```python
from build123d import *

# Parameters (mm, degrees)
SALIENTE_EXTRUIR1_DEPTH = 1
CORTAR_EXTRUIR1_DEPTH   = 0.5
SALIENTE_EXTRUIR2_DEPTH = 0.5


with BuildPart() as part:
    # Croquis1 → Saliente-Extruir1 (new body)
    with BuildSketch(Plane.XY):
        Polygon((0.027506267, 9.99996217), (-9.502029281, 3.116318268), (-5.900083324, -8.073971561), (5.85557725, -8.106307117), (9.519029089, 3.063998239), align=None)
    extrude(amount=SALIENTE_EXTRUIR1_DEPTH)

    # Croquis2 → Cortar-Extruir1 (cut)
    with BuildSketch(Plane.XY.offset(1)):
        Polygon((0.042555256, 9.600245361), (-9.117225611, 3.00711142), (-5.677310567, -7.741748295), (5.608454716, -7.791774999), (9.143526206, 2.926166513), align=None)
    extrude(amount=-CORTAR_EXTRUIR1_DEPTH, mode=Mode.SUBTRACT)

    # Croquis3 → Saliente-Extruir2 (add)
    with BuildSketch(Plane.XY.offset(0.5)):
        Polygon((-5.900083324, -8.073971561), (-0.010506459, -3.819645663), (5.85557725, -8.106307117), (3.629452223, -1.190327659), (9.519029089, 3.063998239), (2.253631293, 3.083982712), (0.027506267, 9.99996217), (-2.236631486, 3.096333795), (-9.502029281, 3.116318268), (-3.635945572, -1.170343186), align=None)
    extrude(amount=SALIENTE_EXTRUIR2_DEPTH)


solid = part.part
```
Check sheet for the modelled part. Datum: model origin and axes. Units: mm. A direction names the side the tool comes from. Coordinates: 2 decimals unless noted, no trailing zeros. Order: outer loops, then holes, each group sorted by start corner. A loop starts at its lowest first (then second) coordinate and runs counter-clockwise, first axis right, second up. Notation, with made-up numbers: (6.25, -13) -> (14.25, -13) arc R19 ccw to (14.25, 5) -> close; hole circle Ø5 at (-10.5, 47.5). An arc over 180 degrees is marked (long way). Write each question's results on one line, items separated by ' | '. Start each with the question number.
1) Section check A-A (z = 0.85). Enter the section's corners in (x, y), and give its area (3 significant figures).
2) Set-up check for faces 5 (the face through (-7.726, -2.4, 0.493)), 6 (the face through (0, -6, 0.5)): record each of +Z, -Z, +X, -X, +Y, -Y from which the full face is reachable in a straight line by a thin tool's end or side.
3) Section check B-B (x = 1.25). Enter the section's corners in (y, z), and give its area (3 significant figures).
4) Material ranges on line 1 along X through (y, z) = (8.75, 0.55); line 2 along X through (y, z) = (-6, 0.8); line 3 along Y through (x, z) = (-3, 0.9), recorded low to high.
5) Depth check by flat-ended pin: pin 1 (2 mm diameter, centred on x = 0, y = -6.5, fed in from +Z). Enter the tip coordinate at first touch or a pass-through.
6) Draft check along Y on faces 1 (the face through (0, -1, 0)), 2 (the face through (7.66, -2.6, 0.49)), 3 (the face through (4, 5, 0.5)), 4 (the face through (2.7, -5.8, 0.7)). Enter one of: pulls with the +Y half, pulls with the -Y half, needs draft (parallel to the pull), parting line crosses it, or undercut.
7) Section check C-C (y = -4.5). Enter the section's corners in (x, z), and give its area (3 significant figures).
8) Section check D-D (x = -1.5). Enter the section's corners in (y, z), and give its area (3 significant figures).
Checked values:
1) outline: (-9.5, 3.12) -> (-5.9, -8.07) -> (5.86, -8.11) -> (9.52, 3.06) -> (0.03, 10) -> close; hole (-9.05, 2.78) -> (-5.73, -7.57) -> (-3.64, -1.17) -> close; hole (-8.97, 3.11) -> (-2.24, 3.1) -> (-0.15, 9.46) -> close; hole (-5.44, -7.74) -> (5.42, -7.79) -> (-0.01, -3.82) -> close; hole (0.19, 9.49) -> (2.25, 3.08) -> (8.95, 3.07) -> close; hole (3.63, -1.19) -> (5.68, -7.57) -> (9.09, 2.75) -> close | area: 131 mm²
2) face 5: +Z, -Z, -X, -Y | face 6: +Z
3) outline: (-8.09, 0) -> (9.11, 0) -> (9.11, 1) -> (8.71, 1) -> (8.71, 0.5) -> (6.2, 0.5) -> (6.2, 1) -> (-4.74, 1) -> (-4.74, 0.5) -> (-7.77, 0.5) -> (-7.77, 1) -> (-8.09, 1) -> close | area: 14.4 mm²
4) line 1: -1.7 to -1.14, -0.38 to 0.43, 1.2 to 1.74 | line 2: -6.57 to -6.23, -5.22 to -3.03, 2.97 to 5.18, 6.2 to 6.55 | line 3: -8.08 to -7.75, -5.98 to 3.1, 7.41 to 7.81
5) pin 1: z = 0.5
6) face 1: needs draft | face 2: pulls with the -Y half | face 3: undercut | face 4: undercut
7) outline: (-7.05, 0) -> (7.04, 0) -> (7.04, 1) -> (6.69, 1) -> (6.69, 0.5) -> (4.69, 0.5) -> (4.69, 1) -> (0.92, 1) -> (0.92, 0.5) -> (-0.95, 0.5) -> (-0.95, 1) -> (-4.73, 1) -> (-4.73, 0.5) -> (-6.71, 0.5) -> (-6.71, 1) -> (-7.05, 1) -> close | area: 11.2 mm²
8) outline: (-8.09, 0) -> (8.9, 0) -> (8.9, 1) -> (8.49, 1) -> (8.49, 0.5) -> (5.34, 0.5) -> (5.34, 1) -> (-4.9, 1) -> (-4.9, 0.5) -> (-7.76, 0.5) -> (-7.76, 1) -> (-8.09, 1) -> close | area: 14.0 mm²
